Verification items for the finished model (mm, model axes). Round coordinates to 2 decimals unless told otherwise and drop trailing zeros. Write each loop counter-clockwise with the first axis right and the second up, starting at its lowest first coordinate (ties: lowest second). Pieces come first, ordered by that corner, then holes. Notation, with made-up numbers: M 84.5,8.25 L 119.5,8.25 A18 ccw 119.5,43.25 Z; hole C 12,-10.75 d6. An arc over 180 degrees is marked long. One line per question, with ' | ' between items.
from build123d import *

# Parameters (mm, degrees)
SKETCH_2_W          = 332.68587988
SKETCH_2_H          = 71.0001569
EXTRUDE_1_DEPTH     = 3
SKETCH_6_R          = 15
CUT_EXTRUDE_1_DEPTH = 10
SKETCH_7_R          = 2.5
CUT_EXTRUDE_2_DEPTH = 10
SKETCH_8_W          = 332.68587988
SKETCH_8_H          = 4.49992155
EXTRUDE_2_DEPTH     = 3
FILLET_1_R          = 10
SKETCH_9_R          = 2.5
CUT_EXTRUDE_3_DEPTH = 308.13402677


with BuildPart() as part:
    # 草图2 → 凸台-拉伸1 (new body)
    with BuildSketch(Plane(origin=(0, 0, 0), x_dir=(1, 0, 0), z_dir=(0, -2.59377104206923e-08, 0.9999999999999998))):
        with Locations((-82.5, -139.998615632)):
            Rectangle(SKETCH_2_W, SKETCH_2_H)
    extrude(amount=EXTRUDE_1_DEPTH)

    # 草图6 → 切除-拉伸1 (cut)
    with BuildSketch(Plane(origin=(0, -7.8e-08, 3), x_dir=(1, 0, 0), z_dir=(0, -2.5937710420692294e-08, 0.9999999999999998))):
        with Locations(Location((-82.5, -139.998615632, 0), (0, 0, 270))):
            Circle(SKETCH_6_R)
    extrude(amount=-CUT_EXTRUDE_1_DEPTH, mode=Mode.SUBTRACT)

    # 草图7 → 切除-拉伸2 (cut)
    with BuildSketch(Plane(origin=(0, 0, 0), x_dir=(-1, 0, 0), z_dir=(0, 2.5937710420692294e-08, -0.9999999999999998))):
        with Locations(Location((238.799997941, -117.998615632, 0), (0, 0, 90))):
            Circle(SKETCH_7_R)
        with Locations(Location((194.799997941, -117.998615632, 0), (0, 0, 90))):
            Circle(SKETCH_7_R)
        with Locations(Location((194.79999794, -161.998615632, 0), (0, 0, 90))):
            Circle(SKETCH_7_R)
        with Locations(Location((238.799997941, -161.998615632, 0), (0, 0, 90))):
            Circle(SKETCH_7_R)
        with Locations(Location((-73.79999794, -161.998615632, 0), (0, 0, 270))):
            Circle(SKETCH_7_R)
        with Locations(Location((-29.79999794, -161.998615632, 0), (0, 0, 270))):
            Circle(SKETCH_7_R)
        with Locations(Location((-29.79999794, -117.998615632, 0), (0, 0, 270))):
            Circle(SKETCH_7_R)
        with Locations(Location((-73.79999794, -117.998615632, 0), (0, 0, 270))):
            Circle(SKETCH_7_R)
    extrude(amount=-CUT_EXTRUDE_2_DEPTH, mode=Mode.SUBTRACT)

    # 草图8 → 凸台-拉伸2 (add)
    with BuildSketch(Plane(origin=(0, -7.8e-08, 3), x_dir=(1, 0, 0), z_dir=(0, -2.5937710420692294e-08, 0.9999999999999998))):
        with Locations((-82.5, -102.248576407)):
            Rectangle(SKETCH_8_W, SKETCH_8_H)
        with Locations((-82.5, -177.748654857)):
            Rectangle(SKETCH_8_W, SKETCH_8_H)
    extrude(amount=-EXTRUDE_2_DEPTH)

    # 圆角1
    fillet_1_edges = [part.edges().sort_by_distance(p)[0] for p in [
        (-248.84293994, -99.998615671, 1.499997406),
        (83.84293994, -99.998615671, 1.499997406),
        (83.84293994, -179.998615671, 1.499995331),
        (-248.84293994, -179.998615671, 1.499995331),
    ]]
    fillet(fillet_1_edges, radius=FILLET_1_R)

    # 草图9 → 切除-拉伸3 (cut, through all)
    with BuildSketch(Plane(origin=(0, 0, 0), x_dir=(-1, 0, 0), z_dir=(0, 2.5937710420692294e-08, -0.9999999999999998))):
        with Locations(Location((202.5, -139.998615632, 0), (0, 0, 90))):
            Circle(SKETCH_9_R)
        with Locations(Location((172.5, -139.998615632, 0), (0, 0, 90))):
            Circle(SKETCH_9_R)
        with Locations(Location((142.5, -139.998615632, 0), (0, 0, 90))):
            Circle(SKETCH_9_R)
        with Locations(Location((112.5, -139.998615632, 0), (0, 0, 90))):
            Circle(SKETCH_9_R)
        with Locations(Location((52.5, -139.998615632, 0), (0, 0, 90))):
            Circle(SKETCH_9_R)
        with Locations(Location((22.5, -139.998615632, 0), (0, 0, 90))):
            Circle(SKETCH_9_R)
        with Locations(Location((-7.5, -139.998615632, 0), (0, 0, 90))):
            Circle(SKETCH_9_R)
        with Locations(Location((-37.5, -139.998615632, 0), (0, 0, 90))):
            Circle(SKETCH_9_R)
        with Locations(Location((-67.5, -139.998615632, 0), (0, 0, 90))):
            Circle(SKETCH_9_R)
        with Locations(Location((232.5, -139.998615632, 0), (0, 0, 90))):
            Circle(SKETCH_9_R)
    extrude(amount=-CUT_EXTRUDE_3_DEPTH, mode=Mode.SUBTRACT)


solid = part.part
1. Thickness scan on line 1 (X direction, y = -164, z = 2.7); line 2 (Y direction, x = 29, z = 1.45); line 3 (X direction, y = -163, z = 0.55). Record the ranges inside material, lowest first.
Results:
line 1: x = -248.84 to -240.3, -237.3 to -196.3, -193.3 to 28.3, 31.3 to 72.3, 75.3 to 83.84 | line 2: y = -180 to -164.37, -159.63 to -120.37, -115.63 to -100 | line 3: x = -248.84 to -241.09, -236.51 to -197.09, -192.51 to 27.51, 32.09 to 71.51, 76.09 to 83.84
2. Section check A-A, the plane y = -132. Record the cut outline in (x, z), then the cut area to 3 significant figures.
Results:
outline: M -248.84,0 L -95.19,0 L -95.19,3 L -248.84,3 Z; M -69.81,0 L 83.84,0 L 83.84,3 L -69.81,3 Z | area: 922 mm2
3. Go/stop test with a flat-tipped pin: P1, Ø8, axis at x = 29.8, y = -118, coming from the +Z side. Record where the tip stops, or that it passes through.
Results:
P1: stops at z = 3
4. Mould release check, pull along Y, two halves, no side actions. Record for faces 1 (the face through (80.991, -176.992, 1.479)), 2 (the face through (-85, -157, 0)), 3 (the face through (-91.627, -128.095, 1.521)): pulls with the +Y half, pulls with the -Y half, needs draft (parallel to the pull), parting line crosses it, or undercut.
Results:
face 1: pulls with the -Y half | face 2: needs draft | face 3: undercut
5. Section check B-B, the plane z = 2.5. Count the separate pieces of the cut face and the enclosed holes in it, then the cut area to 3 significant figures.
Results:
separate pieces: 1 | enclosed holes: 19 | area: 25,500 mm2
